Here's the drawing with two shaded views (mm, measured from the low corner). I have some questions. A direction names the side the tool comes from. Round coordinates to 2 decimals unless told otherwise and drop trailing zeros. Loops run counter-clockwise (first coordinate to the right, second up) from the corner with the lowest first, then second, coordinate; pieces in that order, holes last. Notation, with made-up numbers: (36.25, 81) -> (74.25, 81) arc R34 cw to (74.25, 111) -> close; hole circle Ø2 at (16.5, 86.5). An arc over 180 degrees is marked (long way). Write each question's results on one line, items separated by ' | '. Start each with the question number.
1) For P1, Ø1.2, axis at x = 24, y = 2, coming from the -Z side; P2, Ø1.2, axis at y = 2, z = 30, coming from the -X side; P3, Ø2, axis at x = 27.5, y = 2.5, coming from the +Z side; P4, Ø4.5, axis at x = 21.79, z = 15.61, coming from the +Y side, each with a flat end and sliding along its axis, tell me the tip position at first contact or that it passes through.
2) Which directions (+Z, -Z, +X, -X, +Y, -Y) give clear straight access to the entire face, cutting with the end or side of a thin tool? Please do the marked faces 4, 5, 6 and 7.
3) Imagine slicing it at D-D, the plane x = 8.5. List the corners of the cut face in (y, z) for me, plus the area to 3 significant figures.
4) We'd pull the mould along Z, two halves only. Please class the marked faces 1, 2 and 3: pulls with the +Z half, pulls with the -Z half, needs draft (parallel to the pull), parting line crosses it, or undercut.
5) If I drill on probe 1 along X at (y, z) = (1.1, 15.5) (1 decimal); probe 2 along X at (y, z) = (3.8, 14) (1 decimal); probe 3 along Z at (x, y) = (29.5, 1.65), over which ranges is the centre line in solid material (lowest first)?
6) Imagine slicing it at B-B, the plane z = 17. List the corners of the cut face in (x, y) for me (1 decimal).
7) Imagine slicing it at A-A, the plane x = 17. List the corners of the cut face in (y, z) for me (1 decimal), plus the area to 3 significant figures.
8) Imagine slicing it at C-C, the plane y = 0.75. List the corners of the cut face in (x, z) for me (1 decimal), plus the area to 3 significant figures.
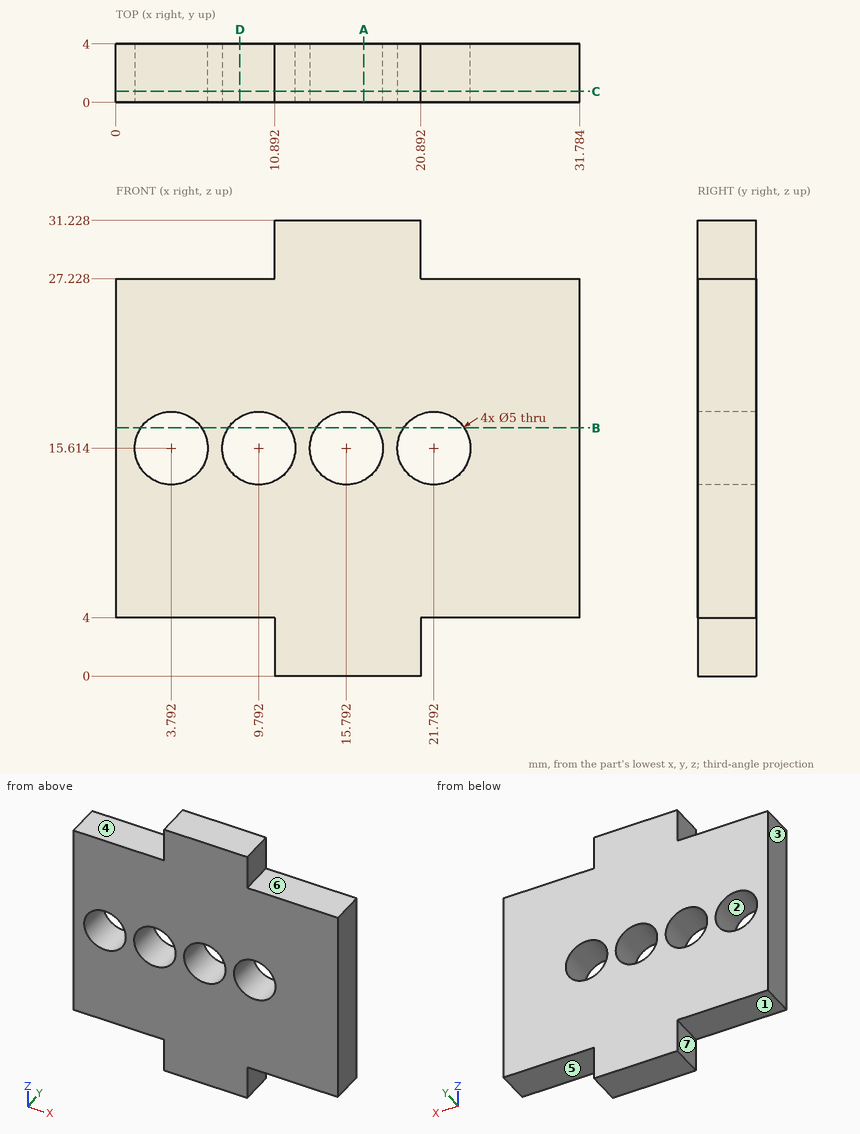
Checked values:
1) P1: z = 4 | P2: x = 10.89 | P3: z = 27.23 | P4: through
2) face 4: +Z, -X, +Y, -Y | face 5: -Z, +X, +Y, -Y | face 6: +Z, +X, +Y, -Y | face 7: -Z, -X, +Y, -Y
3) outline: (0, 4) -> (4, 4) -> (4, 13.47) -> (0, 13.47) -> close; (0, 17.75) -> (4, 17.75) -> (4, 27.23) -> (0, 27.23) -> close | area: 75.8 mm^2
4) face 1: pulls with the -Z half | face 2: undercut | face 3: needs draft
5) probe 1: 0 to 1.3, 6.3 to 7.3, 12.3 to 13.3, 18.3 to 19.3, 24.3 to 31.8 | probe 2: 0 to 1.9, 5.7 to 7.9, 11.7 to 13.9, 17.7 to 19.9, 23.7 to 31.8 | probe 3: 4 to 27.23
6) outline: (0, 0) -> (1.7, 0) -> (1.7, 4) -> (0, 4) -> close; (5.9, 0) -> (7.7, 0) -> (7.7, 4) -> (5.9, 4) -> close; (11.9, 0) -> (13.7, 0) -> (13.7, 4) -> (11.9, 4) -> close; (17.9, 0) -> (19.7, 0) -> (19.7, 4) -> (17.9, 4) -> close; (23.9, 0) -> (31.8, 0) -> (31.8, 4) -> (23.9, 4) -> close
7) outline: (0, 0) -> (4, 0) -> (4, 13.4) -> (0, 13.4) -> close; (0, 17.8) -> (4, 17.8) -> (4, 31.2) -> (0, 31.2) -> close | area: 107 mm^2
8) outline: (0, 4) -> (10.9, 4) -> (10.9, 0) -> (20.9, 0) -> (20.9, 4) -> (31.8, 4) -> (31.8, 27.2) -> (20.9, 27.2) -> (20.9, 31.2) -> (10.9, 31.2) -> (10.9, 27.2) -> (0, 27.2) -> close; hole circle Ø5 at (3.8, 15.6); hole circle Ø5 at (9.8, 15.6); hole circle Ø5 at (15.8, 15.6); hole circle Ø5 at (21.8, 15.6) | area: 740 mm^2
